Here's how the part is built. I have some questions about the finished solid (model axes, mm). A direction names the side the tool comes from. Round coordinates to 2 decimals unless told otherwise and drop trailing zeros. Order: outer loops, then holes, each group sorted by start corner. A loop starts at its lowest first (then second) coordinate and runs counter-clockwise, first axis right, second up. Notation, with made-up numbers: M -25.75,30.25 L -2.75,30.25 A23 cw -2.75,46.25 Z; hole C 48.5,51.25 d9. An arc over 180 degrees is marked long. Write each question's results on one line, items separated by ' | '. Start each with the question number.
```python
from build123d import *
from build123d.topology import SkipClean

# Parameters (mm, degrees)
SKETCH_1_R      = 10
SKETCH_1_R_2    = 1.55
EXTRUDE_1_DEPTH = 2
SKETCH_2_R      = 1.55
EXTRUDE_2_DEPTH = 1
SKETCH_2_3_R    = 1.55
EXTRUDE_3_DEPTH = 2
SKETCH_3_R      = 1.55
SKETCH_3_R_2    = 1
EXTRUDE_5_DEPTH = 1


with BuildPart() as part:
    # Sketch 1 → Extrude 1 (new body)
    with BuildSketch(Plane.XY):
        Circle(SKETCH_1_R)
        Circle(SKETCH_1_R_2, mode=Mode.SUBTRACT)
        with Locations((-7, 0)):
            Circle(SKETCH_1_R_2, mode=Mode.SUBTRACT)
        with Locations((0, 7)):
            Circle(SKETCH_1_R_2, mode=Mode.SUBTRACT)
        with Locations((7, 0)):
            Circle(SKETCH_1_R_2, mode=Mode.SUBTRACT)
        with Locations((0, -7)):
            Circle(SKETCH_1_R_2, mode=Mode.SUBTRACT)
    extrude(amount=EXTRUDE_1_DEPTH)

    # Sketch 2 → Extrude 2 (add)
    # profile 1 of 7: a face of its own
    with BuildSketch(Plane.XY.offset(2)):
        with BuildLine():
            ThreePointArc((-8.719995436, 4.895066864), (-7.404629994, 6.720971258), (-5.714285714, 8.206518066))
            Line((-5.714285714, 8.206518066), (-15.142857143, 1.641303613))
            ThreePointArc((-15.142857143, 1.641303613), (-16, 0), (-15.142857143, -1.641303613))
            Line((-15.142857143, -1.641303613), (-5.714285714, -8.206518066))
            ThreePointArc((-5.714285714, -8.206518066), (-7.404629994, -6.720971258), (-8.719995436, -4.895066864))
            Line((-8.719995436, -4.895066864), (-14.571428571, -0.820651807))
            ThreePointArc((-14.571428571, -0.820651807), (-15, 0), (-14.571428571, 0.820651807))
            Line((-14.571428571, 0.820651807), (-8.719995436, 4.895066864))
        make_face()
    # profile 2 of 7: a face of its own
    with BuildSketch(Plane.XY.offset(2)):
        with BuildLine():
            ThreePointArc((-8.719995436, -4.895066864), (-10, 0), (-8.719995436, 4.895066864))
            Line((-8.719995436, 4.895066864), (-14.571428571, 0.820651807))
            ThreePointArc((-14.571428571, 0.820651807), (-13.53708995, 0.88640526), (-13, 0))
            ThreePointArc((-13, 0), (-13.53708995, -0.88640526), (-14.571428571, -0.820651807))
            Line((-14.571428571, -0.820651807), (-8.719995436, -4.895066864))
        make_face()
    # profile 3 of 7: a face of its own
    with BuildSketch(Plane.XY.offset(2)):
        with BuildLine():
            ThreePointArc((5.714285714, 8.206518066), (0, 10), (-5.714285714, 8.206518066))
            ThreePointArc((-5.714285714, 8.206518066), (-7.404629994, 6.720971258), (-8.719995436, 4.895066864))
            Line((-8.719995436, 4.895066864), (-5.142857143, 7.38586626))
            ThreePointArc((-5.142857143, 7.38586626), (0, 9), (5.142857143, 7.38586626))
            Line((5.142857143, 7.38586626), (8.719995436, 4.895066864))
            ThreePointArc((8.719995436, 4.895066864), (7.404629994, 6.720971258), (5.714285714, 8.206518066))
        make_face()
    # profile 4 of 7: a face of its own
    with BuildSketch(Plane.XY.offset(2)):
        with BuildLine():
            Line((-5.142857143, 7.38586626), (-8.719995436, 4.895066864))
            ThreePointArc((-8.719995436, 4.895066864), (-10, 0), (-8.719995436, -4.895066864))
            Line((-8.719995436, -4.895066864), (-5.142857143, -7.38586626))
            ThreePointArc((-5.142857143, -7.38586626), (0, -9), (5.142857143, -7.38586626))
            Line((5.142857143, -7.38586626), (8.719995436, -4.895066864))
            ThreePointArc((8.719995436, -4.895066864), (9.674708119, -2.529826638), (10, 0))
            ThreePointArc((10, 0), (9.674708119, 2.529826638), (8.719995436, 4.895066864))
            Line((8.719995436, 4.895066864), (5.142857143, 7.38586626))
            ThreePointArc((5.142857143, 7.38586626), (0, 9), (-5.142857143, 7.38586626))
        make_face()
        with Locations((0, -7)):
            Circle(SKETCH_2_R, mode=Mode.SUBTRACT)
        with Locations((-7, 0)):
            Circle(SKETCH_2_R, mode=Mode.SUBTRACT)
        Circle(SKETCH_2_R, mode=Mode.SUBTRACT)
        with Locations((7, 0)):
            Circle(SKETCH_2_R, mode=Mode.SUBTRACT)
        with Locations((0, 7)):
            Circle(SKETCH_2_R, mode=Mode.SUBTRACT)
    # profile 5 of 7: a face of its own
    with BuildSketch(Plane.XY.offset(2)):
        with BuildLine():
            Line((-5.142857143, -7.38586626), (-8.719995436, -4.895066864))
            ThreePointArc((-8.719995436, -4.895066864), (-7.404629994, -6.720971258), (-5.714285714, -8.206518066))
            ThreePointArc((-5.714285714, -8.206518066), (0, -10), (5.714285714, -8.206518066))
            ThreePointArc((5.714285714, -8.206518066), (7.404629994, -6.720971258), (8.719995436, -4.895066864))
            Line((8.719995436, -4.895066864), (5.142857143, -7.38586626))
            ThreePointArc((5.142857143, -7.38586626), (0, -9), (-5.142857143, -7.38586626))
        make_face()
    # profile 6 of 7: a face of its own
    with BuildSketch(Plane.XY.offset(2)):
        with BuildLine():
            Line((15.142857143, 1.641303613), (5.714285714, 8.206518066))
            ThreePointArc((5.714285714, 8.206518066), (7.404629994, 6.720971258), (8.719995436, 4.895066864))
            Line((8.719995436, 4.895066864), (14.571428571, 0.820651807))
            ThreePointArc((14.571428571, 0.820651807), (14.88640526, 0.46291005), (15, 0))
            ThreePointArc((15, 0), (14.88640526, -0.46291005), (14.571428571, -0.820651807))
            Line((14.571428571, -0.820651807), (8.719995436, -4.895066864))
            ThreePointArc((8.719995436, -4.895066864), (7.404629994, -6.720971258), (5.714285714, -8.206518066))
            Line((5.714285714, -8.206518066), (15.142857143, -1.641303613))
            ThreePointArc((15.142857143, -1.641303613), (16, 0), (15.142857143, 1.641303613))
        make_face()
    # profile 7 of 7: a face of its own
    with BuildSketch(Plane.XY.offset(2)):
        with BuildLine():
            Line((14.571428571, 0.820651807), (8.719995436, 4.895066864))
            ThreePointArc((8.719995436, 4.895066864), (9.674708119, 2.529826638), (10, 0))
            ThreePointArc((10, 0), (9.674708119, -2.529826638), (8.719995436, -4.895066864))
            Line((8.719995436, -4.895066864), (14.571428571, -0.820651807))
            ThreePointArc((14.571428571, -0.820651807), (13, 0), (14.571428571, 0.820651807))
        make_face()
    extrude(amount=EXTRUDE_2_DEPTH)

    # Sketch 2_3 → Extrude 3 (add)
    # profile 1 of 3: a face of its own
    with BuildSketch(Plane.XY.offset(2)):
        with BuildLine():
            Line((-5.142857143, 7.38586626), (-8.719995436, 4.895066864))
            ThreePointArc((-8.719995436, 4.895066864), (-10, 0), (-8.719995436, -4.895066864))
            Line((-8.719995436, -4.895066864), (-5.142857143, -7.38586626))
            ThreePointArc((-5.142857143, -7.38586626), (0, -9), (5.142857143, -7.38586626))
            Line((5.142857143, -7.38586626), (8.719995436, -4.895066864))
            ThreePointArc((8.719995436, -4.895066864), (9.674708119, -2.529826638), (10, 0))
            ThreePointArc((10, 0), (9.674708119, 2.529826638), (8.719995436, 4.895066864))
            Line((8.719995436, 4.895066864), (5.142857143, 7.38586626))
            ThreePointArc((5.142857143, 7.38586626), (0, 9), (-5.142857143, 7.38586626))
        make_face()
        with Locations((0, -7)):
            Circle(SKETCH_2_3_R, mode=Mode.SUBTRACT)
        with Locations((-7, 0)):
            Circle(SKETCH_2_3_R, mode=Mode.SUBTRACT)
        Circle(SKETCH_2_3_R, mode=Mode.SUBTRACT)
        with Locations((7, 0)):
            Circle(SKETCH_2_3_R, mode=Mode.SUBTRACT)
        with Locations((0, 7)):
            Circle(SKETCH_2_3_R, mode=Mode.SUBTRACT)
    # profile 2 of 3: a face of its own
    with BuildSketch(Plane.XY.offset(2)):
        with BuildLine():
            ThreePointArc((-8.719995436, -4.895066864), (-10, 0), (-8.719995436, 4.895066864))
            Line((-8.719995436, 4.895066864), (-14.571428571, 0.820651807))
            ThreePointArc((-14.571428571, 0.820651807), (-13.53708995, 0.88640526), (-13, 0))
            ThreePointArc((-13, 0), (-13.53708995, -0.88640526), (-14.571428571, -0.820651807))
            Line((-14.571428571, -0.820651807), (-8.719995436, -4.895066864))
        make_face()
    # profile 3 of 3: a face of its own
    with BuildSketch(Plane.XY.offset(2)):
        with BuildLine():
            Line((14.571428571, 0.820651807), (8.719995436, 4.895066864))
            ThreePointArc((8.719995436, 4.895066864), (9.674708119, 2.529826638), (10, 0))
            ThreePointArc((10, 0), (9.674708119, -2.529826638), (8.719995436, -4.895066864))
            Line((8.719995436, -4.895066864), (14.571428571, -0.820651807))
            ThreePointArc((14.571428571, -0.820651807), (13, 0), (14.571428571, 0.820651807))
        make_face()
    extrude(amount=EXTRUDE_3_DEPTH)

    # Sketch 3 → Extrude 5 (add)
    with SkipClean():  # the faces are left unmerged after this step: merging them gives an invalid solid
        with BuildSketch(Plane.XY.offset(4)):
            with BuildLine():
                Line((15.142857143, 1.641303613), (5.714285714, 8.206518066))
                ThreePointArc((5.714285714, 8.206518066), (0, 10), (-5.714285714, 8.206518066))
                Line((-5.714285714, 8.206518066), (-15.142857143, 1.641303613))
                ThreePointArc((-15.142857143, 1.641303613), (-16, 0), (-15.142857143, -1.641303613))
                Line((-15.142857143, -1.641303613), (-5.714285714, -8.206518066))
                ThreePointArc((-5.714285714, -8.206518066), (0, -10), (5.714285714, -8.206518066))
                Line((5.714285714, -8.206518066), (15.142857143, -1.641303613))
                ThreePointArc((15.142857143, -1.641303613), (16, 0), (15.142857143, 1.641303613))
            make_face()
            with Locations((0, 7)):
                Circle(SKETCH_3_R, mode=Mode.SUBTRACT)
            with Locations((7, 0)):
                Circle(SKETCH_3_R, mode=Mode.SUBTRACT)
            with Locations((0, -7)):
                Circle(SKETCH_3_R, mode=Mode.SUBTRACT)
            Circle(SKETCH_3_R, mode=Mode.SUBTRACT)
            with Locations((-7, 0)):
                Circle(SKETCH_3_R, mode=Mode.SUBTRACT)
            with Locations((-14, 0)):
                Circle(SKETCH_3_R_2, mode=Mode.SUBTRACT)
            with Locations((14, 0)):
                Circle(SKETCH_3_R_2, mode=Mode.SUBTRACT)
        extrude(amount=EXTRUDE_5_DEPTH)


solid = part.part
```
(1) I want a section at B-B on z = 2.4. Write out the boundary of the cut face in (x, y).
(2) I want a section at D-D on y = -7. Write out the boundary of the cut face in (x, z), and give its area (3 significant figures).
(3) I want a section at C-C on x = 7. Write out the boundary of the cut face in (y, z).
(4) Please list where these lines run through material, in increasing order: line 1 (Y direction, x = 0, z = 4.05); line 2 (Y direction, x = 0, z = 3.2); line 3 (Z direction, x = -9, y = 5).
(5) I want a section at A-A on x = 0. Write out the boundary of the cut face in (y, z).
(6) On a 3-axis mill with a long thin cutter (end or side, diameter ignored), from which of +Z, -Z, +X, -X, +Y, -Y can I reach the whole of each face in a straight line? I mean faces 5 (the flat face through (2, 9, 4)), 6 (the flat face through (10.36, -4.97, 4.49)). Say none if no direction works.
(7) If we mould it in two halves opening along Z, with no side actions, what happens to faces 1 (the flat face through (2, 9, 3)), 2 (the flat face through (-10.49, -4.88, 2.49)), 3 (the cylindrical face through (0.1, 9, 3.5)), 4 (the flat face through (0, -2, 5))? For each: pulls with the +Z half, pulls with the -Z half, needs draft (parallel to the pull), parting line crosses it, or undercut.
(8) I'm going to push flat-ended pins straight in: pin 1 Ø1.5 at (x, z) = (-9, 1.5) entering from +Y; pin 2 Ø10 at (x, y) = (3, -1.5) entering from -Z; pin 3 Ø2.5 at (x, y) = (-14, 0) entering from -Z. Where does each tip first touch, or does it pass through?
Solutions:
1) outline: M -15.14,-1.64 L -5.71,-8.21 A10 ccw 5.71,-8.21 L 15.14,-1.64 A2 ccw 15.14,1.64 L 5.71,8.21 A10 ccw -5.71,8.21 L -15.14,1.64 A2 ccw Z; hole C -14,0 d2; hole C -7,0 d3.1; hole C 0,-7 d3.1; hole C 0,0 d3.1; hole C 0,7 d3.1; hole C 7,0 d3.1; hole C 14,0 d2
2) outline: M -7.45,2 L -7.14,2 L -7.14,0 L -1.55,0 L -1.55,5 L -7.45,5 L -7.45,4 L -5.7,4 L -5.7,3 L -7.45,3 Z; M 1.55,0 L 7.14,0 L 7.14,2 L 7.45,2 L 7.45,3 L 5.7,3 L 5.7,4 L 7.45,4 L 7.45,5 L 1.55,5 Z | area: 54.2 mm^2
3) outline: M -7.31,2 L -7.14,2 L -7.14,0 L -1.55,0 L -1.55,5 L -7.31,5 L -7.31,4 L -6.09,4 L -6.09,3 L -7.31,3 Z; M 1.55,0 L 7.14,0 L 7.14,2 L 7.31,2 L 7.31,3 L 6.09,3 L 6.09,4 L 7.31,4 L 7.31,5 L 1.55,5 Z
4) line 1: -10 to -8.55, -5.45 to -1.55, 1.55 to 5.45, 8.55 to 10 | line 2: -9 to -8.55, -5.45 to -1.55, 1.55 to 5.45, 8.55 to 9 | line 3: 2 to 3, 4 to 5
5) outline: M -10,0 L -8.55,0 L -8.55,5 L -10,5 L -10,4 L -9,4 L -9,3 L -10,3 Z; M -5.45,0 L -1.55,0 L -1.55,5 L -5.45,5 Z; M 1.55,0 L 5.45,0 L 5.45,5 L 1.55,5 Z; M 8.55,0 L 10,0 L 10,3 L 9,3 L 9,4 L 10,4 L 10,5 L 8.55,5 Z
6) face 5: none | face 6: +Z, -Z, +X, -Y
7) face 1: undercut | face 2: needs draft | face 3: undercut | face 4: pulls with the +Z half
8) pin 1: y = 6.31 | pin 2: z = 0 | pin 3: z = 2
